Source: three-view drawing plus pictorial views. Frame: mm from the lowest corner of the part. A direction names the side the tool comes from. Coordinates: 2 decimals unless noted, no trailing zeros. Order: outer loops, then holes, each group sorted by start corner. A loop starts at its lowest first (then second) coordinate and runs counter-clockwise, first axis right, second up. Notation, with made-up numbers: (-1.75, 41.25) -> (3.25, 41.25) arc R19 ccw to (3.25, 76.25) -> close; hole circle Ø9 at (39, 35). An arc over 180 degrees is marked (long way). Use one line per item in the form item = value. Start each with the question number.
1) Section query A-A on y = 22.5. Output: boundary loops of the cut face in (x, z), then the cut area to 4 significant figures.
2) Section query B-B on z = 17.25. Output: boundary loops of the cut face in (x, y), then the cut area to 3 significant figures.
3) Access query for the marked faces 1, 2, 3 and 4. Directions: +Z, -Z, +X, -X, +Y, -Y. A direction counts if a zero-diameter tool reaches every point of the face in a straight line with its end or side. Return the directions, or none.
4) Ray query, line 1 along Y through (x, z) = (20, 6.8); line 2 along Z through (x, y) = (1, 31); line 3 along Z through (x, y) = (3.5, 22.5). Return the intervals inside material, ascending.
5) Section query D-D on y = 31. Output: boundary loops of the cut face in (x, z).
6) Draft query along Y for the marked faces 5, 6 and 7. Return one class per face: pulls with the +Y half, pulls with the -Y half, needs draft (parallel to the pull), parting line crosses it, or undercut.
7) Pin query (flat end, axial travel): pin 1 (12 mm diameter, centred on x = 14, z = 17.5, fed in from +Y); pin 2 (7 mm diameter, centred on x = 12.5, z = 13, fed in from -Y); pin 3 (2 mm diameter, centred on y = 10.5, z = 15.5, fed in from +X); pin 4 (1.2 mm diameter, centred on x = 2.5, y = 4.5, fed in from +Z). Return the tip coordinate at first contact, or that it passes through.
8) Section query C-C on x = 4.75. Output: boundary loops of the cut face in (y, z).
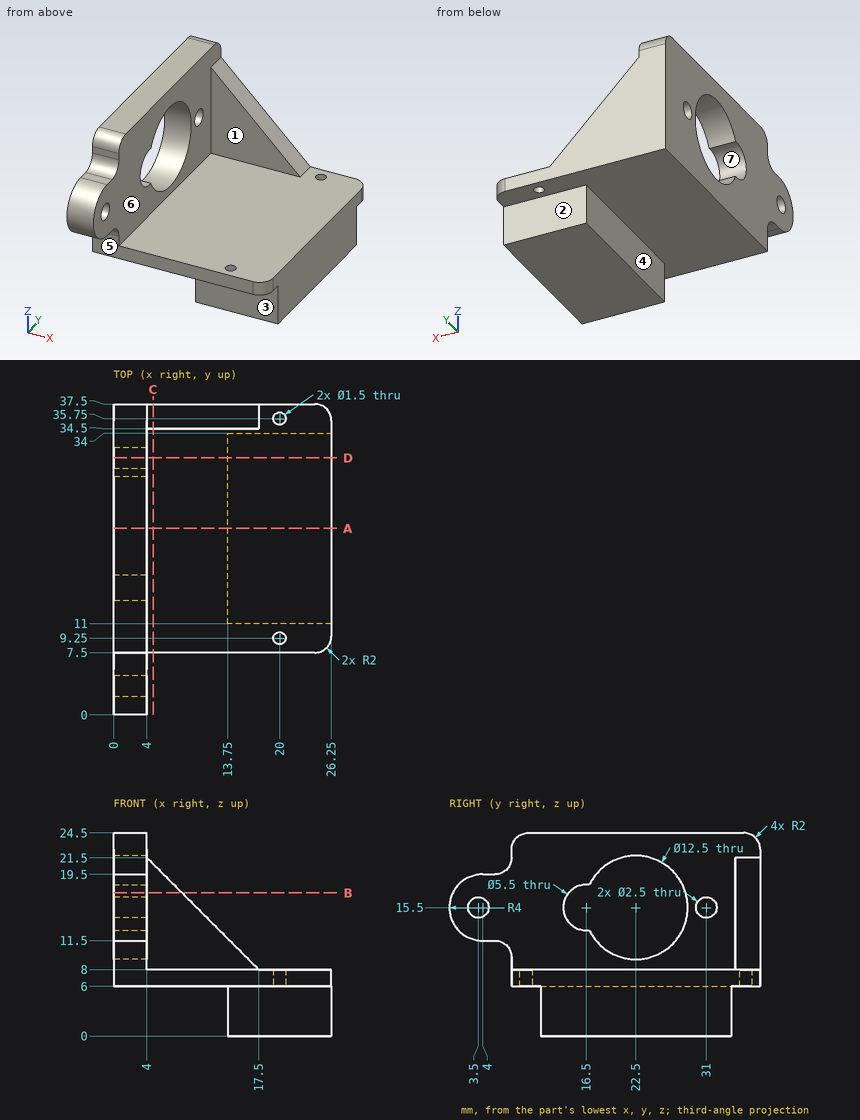
Answers below:
q1.outline = (0, 6) -> (13.75, 6) -> (13.75, 0) -> (26.25, 0) -> (26.25, 8) -> (4, 8) -> (4, 9.25) -> (0, 9.25) -> close; (0, 21.75) -> (4, 21.75) -> (4, 24.5) -> (0, 24.5) -> close
q1.area = 143.5 mm^2
q2.outline = (0, 0.4) -> (4, 0.4) -> (4, 14.38) -> (0, 14.38) -> close; (0, 28.5) -> (4, 28.5) -> (4, 34.5) -> (8.25, 34.5) -> (8.25, 37.5) -> (0, 37.5) -> close
q2.area = 105 mm^2
q3.face_1 = +Z, +X, -Y
q3.face_2 = -Z, +X, -X, +Y
q3.face_3 = -Z, +X, -X, -Y
q3.face_4 = -Z, -X, +Y, -Y
q4.line_1 = 7.5 to 8.5, 10 to 35, 36.5 to 37.5
q4.line_2 = 6 to 14.25, 16.75 to 24.5
q4.line_3 = 6 to 9.25, 21.75 to 24.5
q5.outline = (0, 6) -> (13.75, 6) -> (13.75, 0) -> (26.25, 0) -> (26.25, 8) -> (4, 8) -> (4, 14.25) -> (0, 14.25) -> close; (0, 16.75) -> (4, 16.75) -> (4, 24.5) -> (0, 24.5) -> close
q6.face_5 = pulls with the -Y half
q6.face_6 = needs draft
q6.face_7 = undercut
q7.pin_1 = 37.5
q7.pin_2 = 34.5
q7.pin_3 = 4
q7.pin_4 = 19.5
q8.outline = (7.5, 6) -> (37.5, 6) -> (37.5, 20.75) -> (34.5, 20.75) -> (34.5, 8) -> (7.5, 8) -> close
